Work out the finished part from the listing and answer in its coordinate system (mm). A direction names the side the tool comes from. Give positions to 0.01 mm unless a question says otherwise; leave off trailing zeros. Write each loop counter-clockwise with the first axis right and the second up, starting at its lowest first coordinate (ties: lowest second). Pieces come first, ordered by that corner, then holes.
1) Find section B-B (y = 0.7). Count the separate pieces of the cut face and the enclosed holes in it, plus the area to 3 significant figures.
2) Straight lines are drawn through the part: probe 1 along X at (y, z) = (0.9, 21.5); probe 2 along Z at (x, y) = (-3.5, 0.4); probe 3 along X at (y, z) = (0.45, -19.5). For each, find the intervals that lie inside material, in ascending order.
3) Given pin 1 Ø2.5 at (x, z) = (12.53, -38.66) entering from +Y; pin 2 Ø1 at (x, y) = (-5, 1) entering from +Z, each flat-ended and moving along its own axis, determine where each tip first touches the part or whether it passes through.
4) Find section A-A (z = 26.5). Determine the outline of the cut face in (x, y), plus the area to 3 significant figures.
5) Determine the mould class of faces 1 (the face through (-23.034, 0.986, -10.783)), 2 (the face through (-14.97, 1, -25)) for opening direction X: pulls with the +X half, pulls with the -X half, needs draft (parallel to the pull), parting line crosses it, or undercut.
6) A tool of negligible diameter and unlimited length cuts with its end or side. For faces 3 (the face through (-23.67, 1, 12)), 4 (the face through (16.13, 1, 25)), from which of +Z, -Z, +X, -X, +Y, -Y can it reach the whole face along a straight path? Write none if from no direction.
```python
from build123d import *

# Parameters (mm, degrees)
SKETCH2_R           = 3.5
SKETCH2_R_2         = 1.6
SKETCH2_R_3         = 1.598962018
BOSS_EXTRUDE1_DEPTH = 2


with BuildPart() as part:
    # Sketch2 → Boss-Extrude1 (new body)
    with BuildSketch(Plane(origin=(0, 0, 0), x_dir=(1, 0, 0), z_dir=(0, 1, 0))):
        with BuildLine():
            Line((-23.670097795, -32.056362812), (-23.670097795, 8.618941775))
            ThreePointArc((-23.670097795, 8.618941775), (-23.016737901, 10.809832005), (-21.270097795, 12.285002331))
            ThreePointArc((-21.270097795, 12.285002331), (-20.973864293, 12.401991353), (-20.670097795, 12.497733894))
            Line((-20.670097795, 12.497733894), (-20.670097795, 41.764903086))
            ThreePointArc((-20.670097795, 41.764903086), (-16.675502611, 46.823262428), (-10.828944246, 44.110045668))
            ThreePointArc((-10.828944246, 44.110045668), (-10.464869413, 43.028672598), (-10.420919417, 41.88850305))
            ThreePointArc((-10.420919417, 41.88850305), (-1.470097795, 31.948932783), (7.480723827, 41.88850305))
            ThreePointArc((7.480723827, 41.88850305), (7.524673822, 43.028672598), (7.888748655, 44.110045668))
            ThreePointArc((7.888748655, 44.110045668), (13.735307021, 46.823262428), (17.729902205, 41.764903086))
            Line((17.729902205, 41.764903086), (17.729902205, 12.497733894))
            ThreePointArc((17.729902205, 12.497733894), (18.033668702, 12.401991353), (18.329902205, 12.285002331))
            ThreePointArc((18.329902205, 12.285002331), (20.076542311, 10.809832005), (20.729902205, 8.618941775))
            Line((20.729902205, 8.618941775), (20.729902205, -32.056362812))
            ThreePointArc((20.729902205, -32.056362812), (21.209983868, -38.107008106), (22.164905513, -44.10108114))
            ThreePointArc((22.164905513, -44.10108114), (-1.470097795, -61.389315795), (-25.105101104, -44.10108114))
            ThreePointArc((-25.105101104, -44.10108114), (-24.150179459, -38.107008106), (-23.670097795, -32.056362812))
        make_face()
        with Locations(Location((-1.470097795, -54.218974573, 0), (0, 0, 270))):
            Circle(SKETCH2_R, mode=Mode.SUBTRACT)
        with Locations(Location((7.629909443, -51.858302161, 0), (0, 0, 270))):
            Circle(SKETCH2_R, mode=Mode.SUBTRACT)
        with Locations(Location((-10.570105034, -51.858302161, 0), (0, 0, 270))):
            Circle(SKETCH2_R, mode=Mode.SUBTRACT)
        with Locations(Location((-19.470097795, -44.839315795, 0), (0, 0, 270))):
            Circle(SKETCH2_R_2, mode=Mode.SUBTRACT)
        with Locations(Location((16.529902205, -44.839315795, 0), (0, 0, 270))):
            Circle(SKETCH2_R_2, mode=Mode.SUBTRACT)
        with Locations(Location((-19.470097795, 8.160684205, 0), (0, 0, 270))):
            Circle(SKETCH2_R_2, mode=Mode.SUBTRACT)
        with Locations(Location((16.529902205, 8.160684205, 0), (0, 0, 270))):
            Circle(SKETCH2_R_2, mode=Mode.SUBTRACT)
        with Locations(Location((-15.470097795, 38.660684205, 0), (0, 0, 270))):
            Circle(SKETCH2_R_3, mode=Mode.SUBTRACT)
        with Locations(Location((12.529902205, 38.660684205, 0), (0, 0, 270))):
            Circle(SKETCH2_R_3, mode=Mode.SUBTRACT)
        with BuildLine():
            Line((-16.970097795, 31.660684205), (-16.970097795, 18.660684205))
            ThreePointArc((-16.970097795, 18.660684205), (-15.970097795, 17.660684205), (-14.970097795, 18.660684205))
            Line((-14.970097795, 18.660684205), (-14.970097795, 31.660684205))
            ThreePointArc((-14.970097795, 31.660684205), (-15.970097795, 32.660684205), (-16.970097795, 31.660684205))
        make_face(mode=Mode.SUBTRACT)
        with BuildLine():
            Line((12.029902205, 31.660684205), (12.029902205, 18.660684205))
            ThreePointArc((12.029902205, 18.660684205), (13.029902205, 17.660684205), (14.029902205, 18.660684205))
            Line((14.029902205, 18.660684205), (14.029902205, 31.660684205))
            ThreePointArc((14.029902205, 31.660684205), (13.029902205, 32.660684205), (12.029902205, 31.660684205))
        make_face(mode=Mode.SUBTRACT)
        with BuildLine():
            Line((13.729902205, -9.839315795), (13.729902205, -38.839315795))
            ThreePointArc((13.729902205, -38.839315795), (14.022795424, -39.546422576), (14.729902205, -39.839315795))
            Line((14.729902205, -39.839315795), (15.129902205, -39.839315795))
            ThreePointArc((15.129902205, -39.839315795), (15.837008986, -39.546422576), (16.129902205, -38.839315795))
            Line((16.129902205, -38.839315795), (16.129902205, -9.839315795))
            ThreePointArc((16.129902205, -9.839315795), (15.837008986, -9.132209013), (15.129902205, -8.839315795))
            Line((15.129902205, -8.839315795), (14.729902205, -8.839315795))
            ThreePointArc((14.729902205, -8.839315795), (14.022795424, -9.132209013), (13.729902205, -9.839315795))
        make_face(mode=Mode.SUBTRACT)
        with BuildLine():
            Line((-16.670097795, -9.839315795), (-16.670097795, -38.839315795))
            ThreePointArc((-16.670097795, -38.839315795), (-16.962991014, -39.546422576), (-17.670097795, -39.839315795))
            Line((-17.670097795, -39.839315795), (-18.070097795, -39.839315795))
            ThreePointArc((-18.070097795, -39.839315795), (-18.777204576, -39.546422576), (-19.070097795, -38.839315795))
            Line((-19.070097795, -38.839315795), (-19.070097795, -9.839315795))
            ThreePointArc((-19.070097795, -9.839315795), (-18.777204576, -9.132209013), (-18.070097795, -8.839315795))
            Line((-18.070097795, -8.839315795), (-17.670097795, -8.839315795))
            ThreePointArc((-17.670097795, -8.839315795), (-16.962991014, -9.132209013), (-16.670097795, -9.839315795))
        make_face(mode=Mode.SUBTRACT)
        with BuildLine():
            Line((-9.070097795, 24.660684205), (9.529902205, 24.660684205))
            ThreePointArc((9.529902205, 24.660684205), (10.237008986, 24.953577424), (10.529902205, 25.660684205))
            Line((10.529902205, 25.660684205), (10.529902205, 26.660684205))
            ThreePointArc((10.529902205, 26.660684205), (10.237008986, 27.367790987), (9.529902205, 27.660684205))
            Line((9.529902205, 27.660684205), (-9.070097795, 27.660684205))
            ThreePointArc((-9.070097795, 27.660684205), (-9.777204576, 27.367790987), (-10.070097795, 26.660684205))
            Line((-10.070097795, 26.660684205), (-10.070097795, 25.660684205))
            ThreePointArc((-10.070097795, 25.660684205), (-9.777204576, 24.953577424), (-9.070097795, 24.660684205))
        make_face(mode=Mode.SUBTRACT)
        with BuildLine():
            Line((-9.070097795, -5.339315795), (9.529902205, -5.339315795))
            ThreePointArc((9.529902205, -5.339315795), (10.237008986, -5.046422576), (10.529902205, -4.339315795))
            Line((10.529902205, -4.339315795), (10.529902205, -3.339315795))
            ThreePointArc((10.529902205, -3.339315795), (10.237008986, -2.632209013), (9.529902205, -2.339315795))
            Line((9.529902205, -2.339315795), (-9.070097795, -2.339315795))
            ThreePointArc((-9.070097795, -2.339315795), (-9.777204576, -2.632209013), (-10.070097795, -3.339315795))
            Line((-10.070097795, -3.339315795), (-10.070097795, -4.339315795))
            ThreePointArc((-10.070097795, -4.339315795), (-9.777204576, -5.046422576), (-9.070097795, -5.339315795))
        make_face(mode=Mode.SUBTRACT)
        with BuildLine():
            ThreePointArc((11.592409226, 2.277082303), (8.483157974, 8.222231222), (2.638014207, 11.51563878))
            ThreePointArc((2.638014207, 11.51563878), (2.121996842, 11.817028658), (1.869995807, 12.358882197))
            add(Edge.make_bspline(
                [(1.869995807, 12.358882197), (1.842662891, 12.564920807), (1.645816717, 13.772533118), (0.643080373, 16.073708791), (-1.324607952, 18.345688068), (-3.18934686, 19.343792608), (-3.972407265, 19.727563494), (-4.154351902, 19.815161669)],
                knots=[1.415793745, 1.415793745, 1.415793745, 1.415793745, 2.040258905, 5.097099775, 8.794778711, 10.800795525, 11.405761141, 11.405761141, 11.405761141, 11.405761141], degree=3))
            ThreePointArc((-4.154351902, 19.815161669), (-4.506981756, 20.541481709), (-3.880471106, 21.050768485))
            add(Edge.make_bspline(
                [(12.880043513, 2.387180569), (12.881065186, 2.430898093), (12.88208686, 2.474615617), (12.883108534, 2.518333141), (12.918901743, 4.049928037), (13.017697673, 8.277415536), (10.28287236, 14.599600939), (4.282341197, 19.709461541), (-0.897163555, 21.050696374), (-3.734485369, 21.052584871), (-3.880471106, 21.050768485)],
                knots=[-0.130629719, -0.130629719, -0.130629719, -0.130629719, 0, 0, 0, 4.576467099, 12.631902537, 19.61060331, 27.611731203, 28.045840496, 28.045840496, 28.045840496, 28.045840496], degree=3))
            ThreePointArc((12.880043513, 2.387180569), (12.285596676, 1.754729973), (11.592409226, 2.277082303))
        make_face(mode=Mode.SUBTRACT)
        with BuildLine():
            ThreePointArc((-1.689370597, 11.692522502), (-5.997136857, 10.178575784), (-9.409048266, 7.14414909))
            ThreePointArc((-9.409048266, 7.14414909), (-9.907398641, 6.794332332), (-10.516256933, 6.79838691))
            add(Edge.make_bspline(
                [(-9.073047111, 20.195403041), (-9.924041196, 19.924818402), (-11.457295922, 19.314866074), (-13.88656058, 17.968625132), (-15.738010724, 15.472586344), (-15.963993383, 12.140965148), (-14.831238886, 9.284075293), (-12.803522888, 7.546235802), (-11.333770861, 7.065682842), (-10.715557595, 6.86355064), (-10.649124041, 6.841829396), (-10.582690487, 6.820108153), (-10.516256933, 6.79838691)],
                knots=[33.27876941, 33.27876941, 33.27876941, 33.27876941, 35.932769732, 38.174441101, 41.572939786, 44.716597805, 47.793369971, 50.469296473, 52.412006936, 52.412006936, 52.412006936, 52.620771722, 52.620771722, 52.620771722, 52.620771722], degree=3))
            ThreePointArc((-9.073047111, 20.195403041), (-8.762207832, 20.242386416), (-8.452141885, 20.190544322))
            add(Edge.make_bspline(
                [(-0.856220767, 12.89935179), (-0.919315201, 13.18303538), (-1.361040524, 14.788219391), (-3.220498182, 16.995304302), (-5.690570357, 19.103609418), (-7.513737765, 19.869024907), (-8.35180533, 20.156903184), (-8.452141885, 20.190544322)],
                knots=[1.628367635, 1.628367635, 1.628367635, 1.628367635, 2.502760397, 6.666081456, 9.886557607, 12.220662199, 12.537412771, 12.537412771, 12.537412771, 12.537412771], degree=3))
            ThreePointArc((-0.856220767, 12.89935179), (-1.009428131, 12.114118033), (-1.689370597, 11.692522502))
        make_face(mode=Mode.SUBTRACT)
    extrude(amount=BOSS_EXTRUDE1_DEPTH)


solid = part.part
```
Results:
1. separate pieces: 1
1. enclosed holes: 17
1. area: 3,460 mm2
2. probe 1: x = -23.67 to -19.07, -16.67 to 13.73, 16.13 to 20.73
2. probe 2: z = -32.18 to -27.66, -24.66 to -21.05, -19.49 to -17.13, -11.28 to 2.34, 5.34 to 51.37, 57.07 to 61.31
2. probe 3: x = -20.67 to -16.97, -14.97 to -10.92, -6.71 to -3.51, 3.39 to 12.03, 14.03 to 17.73
3. pin 1: passes through
3. pin 2: stops at z = 61.2
4. outline: (-23.67, 0) - (-19.07, 0) - (-19.07, 2) - (-23.67, 2) - close; (-16.67, 0) - (13.73, 0) - (13.73, 2) - (-16.67, 2) - close; (16.13, 0) - (20.73, 0) - (20.73, 2) - (16.13, 2) - close
4. area: 79.2 mm2
5. face 1: pulls with the -X half
5. face 2: undercut
6. face 3: -Z, -X, +Y, -Y
6. face 4: +Y, -Y
